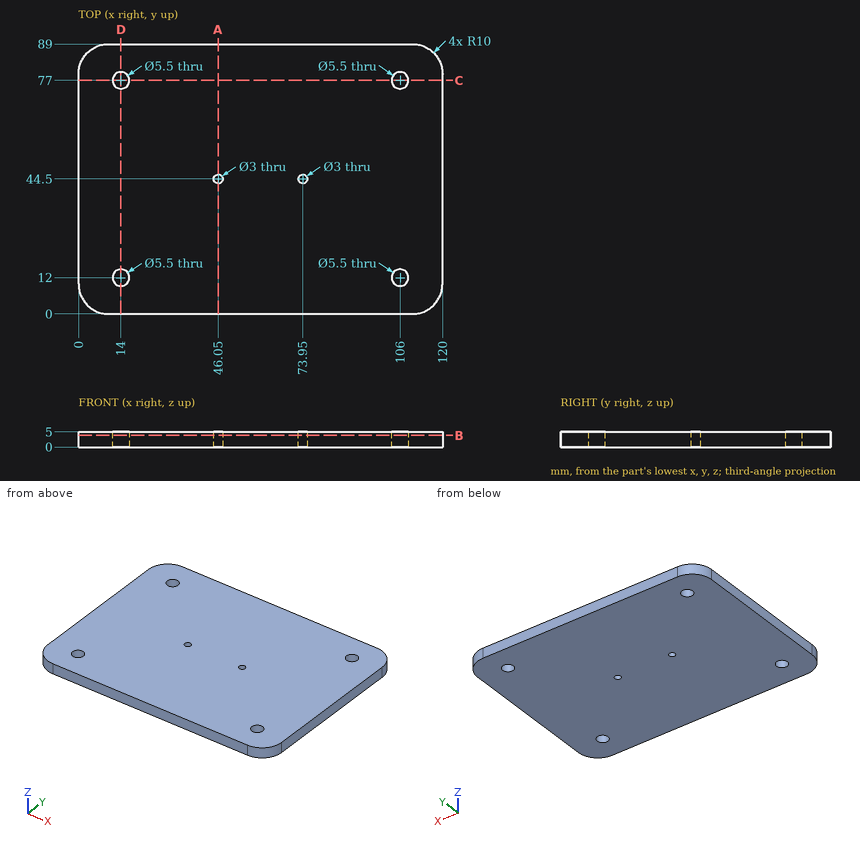
Answer from the drawing. Dimensions are ordinates in mm from the lowest x, y and z of the part. Give positions to 0.01 mm unless a question says otherwise; leave off trailing zeros. Order: outer loops, then holes, each group sorted by start corner. A loop starts at its lowest first (then second) coordinate and runs counter-clockwise, first axis right, second up. Notation, with made-up numbers: (64, 39) - (108, 39) arc R25 cw to (108, 77) - close; hole circle Ø10 at (72, 37). An arc over 180 degrees is marked (long way). One line per item, written item: value. Start each with the question number.
1) Find the intervals of material crossed by L1, parallel to Y at x = 14, z = 1.2; L2, parallel to Y at x = 46.05, z = 2.5; L3, parallel to X at y = 77, z = 3, in increasing order.
2) A cutting plane is placed at B-B on z = 3.9. Give the vertices of the cut face in (x, y).
3) A cutting plane is placed at C-C on y = 77. Give the vertices of the cut face in (x, z).
4) Given pin 1 Ø4 at (x, y) = (101.5, 38.5) entering from -Z; pin 2 Ø2.5 at (x, y) = (73.95, 44.5) entering from +Z, each flat-ended and moving along its own axis, determine where each tip first touches the part or whether it passes through.
5) A cutting plane is placed at D-D on x = 14. Give the vertices of the cut face in (y, z), then the cut area to 3 significant figures.
6) A cutting plane is placed at A-A on x = 46.05. Give the vertices of the cut face in (y, z).
Answer sheet:
1. L1: y = 0 to 9.25, 14.75 to 74.25, 79.75 to 89
1. L2: y = 0 to 43, 46 to 89
1. L3: x = 0 to 11.25, 16.75 to 103.25, 108.75 to 120
2. outline: (0, 10) arc R10 ccw to (10, 0) - (110, 0) arc R10 ccw to (120, 10) - (120, 79) arc R10 ccw to (110, 89) - (10, 89) arc R10 ccw to (0, 79) - close; hole circle Ø5.5 at (14, 12); hole circle Ø5.5 at (14, 77); hole circle Ø3 at (46.05, 44.5); hole circle Ø3 at (73.95, 44.5); hole circle Ø5.5 at (106, 12); hole circle Ø5.5 at (106, 77)
3. outline: (0, 0) - (11.25, 0) - (11.25, 5) - (0, 5) - close; (16.75, 0) - (103.25, 0) - (103.25, 5) - (16.75, 5) - close; (108.75, 0) - (120, 0) - (120, 5) - (108.75, 5) - close
4. pin 1: stops at z = 0
4. pin 2: passes through
5. outline: (0, 0) - (9.25, 0) - (9.25, 5) - (0, 5) - close; (14.75, 0) - (74.25, 0) - (74.25, 5) - (14.75, 5) - close; (79.75, 0) - (89, 0) - (89, 5) - (79.75, 5) - close
5. area: 390 mm2
6. outline: (0, 0) - (43, 0) - (43, 5) - (0, 5) - close; (46, 0) - (89, 0) - (89, 5) - (46, 5) - close
